For this review, take the finished solid that the model builds, in its own axes (mm). A direction names the side the tool comes from. Give positions to 0.01 mm unless a question says otherwise; leave off trailing zeros. Order: outer loops, then holes, each group sorted by start corner. A loop starts at its lowest first (then second) coordinate and runs counter-clockwise, first axis right, second up.
Item 1: The part is to be moulded in two halves that separate along Y. For faces 3 (the flat face through (0, 10, 7)), 4 (the cylindrical face through (-0.1, 2.75, 7.4)), 5 (the flat face through (-10, 0, 7)), say which applies: released by +Y, released by -Y, zero draft, split by the parting line, or undercut.
Item 2: Consider section B-B (x = 0). Give the boundary of the cut face in (y, z).
Item 3: For probe 1 along X at (y, z) = (0, 6.75); probe 2 along Y at (x, z) = (0, 6.75); probe 3 along X at (y, z) = (1.5, 4), list the stretches that pass through material, from the lowest coordinate up.
Item 4: Machinability: for faces 1 (the flat face through (0, -2.25, 7)), 2 (the flat face through (-4, 0, 15)), which of the approach directions +Z, -Z, +X, -X, +Y, -Y give a long, thin tool a straight path to every point of the face, cutting with its end or side? Answer none if there is none.
Item 5: Consider section A-A (z = 8). Give the boundary of the cut face in (x, y), plus the area to 3 significant figures.
```python
from build123d import *

# Parameters (mm, degrees)
ESQUISSE1_W        = 20
ESQUISSE1_H        = 20
BOSS_EXTRU_1_DEPTH = 15
CONG_1_R           = 0.5


with BuildPart() as part:
    # Esquisse1 → Boss.-Extru.1 (new body)
    with BuildSketch(Plane.XY):
        Rectangle(ESQUISSE1_W, ESQUISSE1_H)
        with BuildLine():
            Line((1.58113883, -2.25), (-1.58113883, -2.25))
            ThreePointArc((-1.58113883, -2.25), (0, 2.75), (1.58113883, -2.25))
        make_face(mode=Mode.SUBTRACT)
    extrude(amount=BOSS_EXTRU_1_DEPTH)

    # Congé1
    cong_1_edges = [part.edges().sort_by_distance(p)[0] for p in [
        (0, -2.25, 0),
        (0, 2.75, 0),
        (0, -2.25, 15),
        (-10, -10, 7.5),
        (-10, 10, 7.5),
        (10, 10, 7.5),
        (10, -10, 7.5),
        (0, -10, 15),
        (10, 0, 15),
        (0, 10, 15),
        (-10, 0, 15),
        (0, 2.75, 15),
        (-10, 0, 0),
        (0, 10, 0),
        (10, 0, 0),
        (0, -10, 0),
    ]]
    fillet(cong_1_edges, radius=CONG_1_R)


solid = part.part
```
Resolved:
1. face 3: released by +Y
1. face 4: undercut
1. face 5: zero draft
2. outline: (-10, 0.5) arc R0.5 ccw to (-9.5, 0) - (-2.75, 0) arc R0.5 ccw to (-2.25, 0.5) - (-2.25, 14.5) arc R0.5 ccw to (-2.75, 15) - (-9.5, 15) arc R0.5 ccw to (-10, 14.5) - close; (2.75, 0.5) arc R0.5 ccw to (3.25, 0) - (9.5, 0) arc R0.5 ccw to (10, 0.5) - (10, 14.5) arc R0.5 ccw to (9.5, 15) - (3.25, 15) arc R0.5 ccw to (2.75, 14.5) - close
3. probe 1: x = -10 to -2.75, 2.75 to 10
3. probe 2: y = -10 to -2.25, 2.75 to 10
3. probe 3: x = -10 to -2.3, 2.3 to 10
4. face 1: +Z, -Z
4. face 2: +Z, +X, -X, +Y, -Y
5. outline: (-10, -9.5) arc R0.5 ccw to (-9.5, -10) - (9.5, -10) arc R0.5 ccw to (10, -9.5) - (10, 9.5) arc R0.5 ccw to (9.5, 10) - (-9.5, 10) arc R0.5 ccw to (-10, 9.5) - close; hole (-1.58, -2.25) - (1.58, -2.25) arc R2.75 ccw (long way) to start
5. area: 377 mm2
